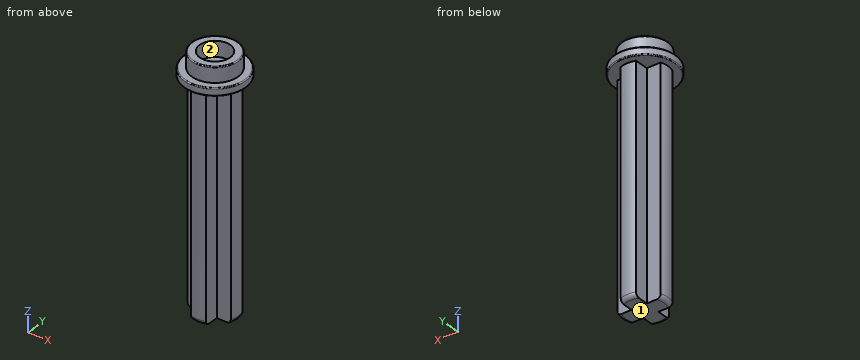
Autodesk Inventor part; units mm, degrees
ref_plane "YZ Plane" through (0, 0, 0) normal (1, 0, 0) x (0, 1, 0)
ref_plane "XZ Plane" through (0, 0, 0) normal (0, 1, 0) x (-1, 0, 0)
ref_plane "XY Plane" through (0, 0, 0) normal (0, 0, 1) x (1, 0, 0)
sketch "Sketch1" plane through (0, 0, 0) normal (0, 0, 1) x (1, 0, 0)
  circle A0 centre (0, 0) radius 2.4 construction
  line L0 (-0.8, 2.2627) -> (-0.8, 0.8)
  line L1 (-0.8, 0.8) -> (-2.2627, 0.8)
  line L2 (-2.2627, -0.8) -> (-0.8, -0.8)
  line L3 (-0.8, -0.8) -> (-0.8, -2.2627)
  line L4 (0.8, -2.2627) -> (0.8, -0.8)
  line L5 (0.8, -0.8) -> (2.2627, -0.8)
  line L6 (2.2627, 0.8) -> (0.8, 0.8)
  line L7 (0.8, 0.8) -> (0.8, 2.2627)
  arc A1 (0.8, 2.2627) -> (-0.8, 2.2627) centre (0, 0) ccw
  arc A2 (-2.2627, 0.8) -> (-2.2627, -0.8) centre (0, 0) ccw
  arc A3 (-0.8, -2.2627) -> (0.8, -2.2627) centre (0, 0) ccw
  arc A4 (2.2627, -0.8) -> (2.2627, 0.8) centre (0, 0) ccw
  dimension "d0" = 4.8
  dimension "d1" = 1.6
extrude "Extrusion1" add sketch "Sketch1" along normal mid plane 23.2
sketch "Sketch2" plane through (0, 0, 11.6) normal (0, 0, 1) x (1, 0, 0)
  arc A0 (0.8, 2.2627) -> (-0.8, 2.2627) centre (0, 0) ccw
  circle A1 centre (0, 0) radius 3.2
  dimension "d7" = 6.4
extrude "Extrusion2" add sketch "Sketch2" along normal blind 0.8
sketch "Sketch3" plane through (0, 0, 12.4) normal (0, 0, 1) x (1, 0, 0)
  circle A0 centre (0, 0) radius 3.2
  circle A1 centre (0, 0) radius 2.4
  circle A2 centre (0, 0) radius 1.6
  dimension "d10" = 4.8
  dimension "d11" = 3.2
extrude "Extrusion3" add sketch "Sketch3" along normal blind 1.6 contours A1
sketch3d "Sketch4"
feature "LEGO_SM:1" [suppressed]
fillet "Fillet1" radius 0.4 4 edges at (2.4, 0, -11.6) (0, 2.4, -11.6) (-2.4, 0, -11.6) (0, -2.4, -11.6)
fillet "Fillet1" radius 0.1 3 edges at (-2.4, 0, 14) (-3.2, 0, 12.4) (-3.2, 0, 11.6)
equation "\"d0\" = kd"
equation "\"d1\" = axlet"
equation "\"d2\" = 3 * lu - tsl"
equation "\"d7\" = tsd"
equation "\"d8\" = tsl"
equation "\"d10\" = kd"
equation "\"d11\" = rd"
equation "\"d12\" = knobh"
equation "\"d4\" = tf"
equation "\"d14\" = lf"
equation "\"lf\" = 0.1"
equation "\"tf\" = 0.4"
properties part number "6587-DkTan" material "ABS Plastic"
Part model, mm, in its own coordinate system. Face numbers are marked on the shaded views. Coordinates: 2 decimals unless noted, no trailing zeros. Write each loop counter-clockwise with the first axis right and the second up, starting at its lowest first coordinate (ties: lowest second). Pieces come first, ordered by that corner, then holes. Notation, with made-up numbers: (58, 22) - (100, 22) arc R8 cw to (100, 33) - close; hole circle Ø3 at (64.5, 80). An arc over 180 degrees is marked (long way). Put each result on its own line as item: value.
1. Flat gauge pins, fed straight in: pin 1 Ø2 at (x, z) = (-2, 10.5) entering from -Y; pin 2 Ø0.7 at (y, z) = (-2, 2) entering from +X; pin 3 Ø1.6 at (x, z) = (1.5, -2) entering from +Y. Where does each tip first touch, or does it go through?
Final values:
pin 1: stops at y = -0.8
pin 2: stops at x = 0.8
pin 3: stops at y = 2.3
2. Probe line 1 along Y through (x, z) = (0, 13.4); line 2 along X through (y, z) = (1.5, -2.75); line 3 along Z through (x, y) = (2.5, 0.5). List the from-to ranges inside material, lowest first. Write a range as [from, to].
Final values:
line 1: y = [-2.4, -1.6], [1.6, 2.4]
line 2: x = [-0.8, 0.8]
line 3: z = [11.6, 12.4]
3. Two-plate mould, pull along X, no slides. Class the marked faces 1 and 2: +X half, -X half, draft (parallel to the pull), parting line (faces both ways), or undercut.
Final values:
face 1: draft
face 2: undercut
4. Band-saw the part on A-A (z = 7). Write the cut outline in (x, y).
Final values:
outline: (-2.26, -0.8) - (-0.8, -0.8) - (-0.8, -2.26) arc R2.4 ccw to (0.8, -2.26) - (0.8, -0.8) - (2.26, -0.8) arc R2.4 ccw to (2.26, 0.8) - (0.8, 0.8) - (0.8, 2.26) arc R2.4 ccw to (-0.8, 2.26) - (-0.8, 0.8) - (-2.26, 0.8) arc R2.4 ccw to start
5. Band-saw the part on B-B (y = 0). Write the cut outline in (x, z).
Final values:
outline: (-3.2, 11.7) arc R0.1 ccw to (-3.1, 11.6) - (-2.4, 11.6) - (-2.4, -11.2) arc R0.4 ccw to (-2, -11.6) - (2, -11.6) arc R0.4 ccw to (2.4, -11.2) - (2.4, 11.6) - (3.1, 11.6) arc R0.1 ccw to (3.2, 11.7) - (3.2, 12.3) arc R0.1 ccw to (3.1, 12.4) - (2.4, 12.4) - (2.4, 13.9) arc R0.1 ccw to (2.3, 14) - (1.6, 14) - (1.6, 12.4) - (-1.6, 12.4) - (-1.6, 14) - (-2.3, 14) arc R0.1 ccw to (-2.4, 13.9) - (-2.4, 12.4) - (-3.1, 12.4) arc R0.1 ccw to (-3.2, 12.3) - close
